Source: CAD feature listing. Evaluate the final solid. Frame: model axes, mm. Give positions to 0.01 mm unless a question says otherwise; leave off trailing zeros. Order: outer loops, then holes, each group sorted by start corner. A loop starts at its lowest first (then second) coordinate and runs counter-clockwise, first axis right, second up. Notation, with made-up numbers: (-14, 8.5) - (31, 8.5) arc R23 cw to (31, 43.5) - close; hole circle Ø1 at (-23, 60). An arc over 180 degrees is marked (long way). Answer as CSV lines item,"result".
```python
from build123d import *

# Parameters (mm, degrees)
SKETCH_1_R          = 1.621125
EXTRUDE_700_DEPTH   = 65
SKETCH_2_OUTSIDE_W  = 249.76
SKETCH_2_OUTSIDE_H  = 250.688
SKETCH_2_OUTSIDE_R  = 3
CUT_EXTRUDE_1_DEPTH = 66
CUT_EXTRUDE_1_TAPER = 60
SKETCH_3_OUTSIDE_W  = 249.76
SKETCH_3_OUTSIDE_H  = 250.688
SKETCH_3_OUTSIDE_R  = 3
CUT_EXTRUDE_2_DEPTH = 66
CUT_EXTRUDE_2_TAPER = 60


with BuildPart() as part:
    # 草图1 → Extrude 700 (new body)
    with BuildSketch(Plane.XY):
        Polygon((0, 3.464101615), (-3, 1.732050808), (-3, -1.732050808), (0, -3.464101615), (3, -1.732050808), (3, 1.732050808), align=None)
        Circle(SKETCH_1_R, mode=Mode.SUBTRACT)
    extrude(amount=EXTRUDE_700_DEPTH)

    # 草图2 outside → 切除-拉伸1 (cut, through all)
    with BuildSketch(Plane(origin=(0, 0, 0), x_dir=(-1, 0, 0), z_dir=(0, 0, -1))):
        Rectangle(SKETCH_2_OUTSIDE_W, SKETCH_2_OUTSIDE_H)
        Circle(SKETCH_2_OUTSIDE_R, mode=Mode.SUBTRACT)
    extrude(amount=-CUT_EXTRUDE_1_DEPTH, taper=CUT_EXTRUDE_1_TAPER, mode=Mode.SUBTRACT)

    # 草图3 outside → 切除-拉伸2 (cut, through all)
    with BuildSketch(Plane.XY.offset(65)):
        Rectangle(SKETCH_3_OUTSIDE_W, SKETCH_3_OUTSIDE_H)
        Circle(SKETCH_3_OUTSIDE_R, mode=Mode.SUBTRACT)
    extrude(amount=-CUT_EXTRUDE_2_DEPTH, taper=CUT_EXTRUDE_2_TAPER, mode=Mode.SUBTRACT)


solid = part.part
```
(1) Mould query, pull axis X, two halves, no side actions, for faces 1 (the conical face through (-2.744, 1.575, 64.905)), 2 (the flat face through (1.3, -1.3, 65)), 3 (the cylindrical face through (-0.351, -1.583, 32.045)). Classes: released by +X, released by -X, zero draft, split by the parting line, or undercut.
Completed:
face 1,"released by -X"
face 2,"zero draft"
face 3,"undercut"
(2) Ray query, line 1 (Y direction, x = 0, z = 27); line 2 (Y direction, x = 0.25, z = 38); line 3 (X direction, y = 0.75, z = 40). Return the intervals inside material, ascending. Write a range as from..to.
Completed:
line 1,"-3.46..-1.62, 1.62..3.46"
line 2,"-3.32..-1.6, 1.6..3.32"
line 3,"-3..-1.44, 1.44..3"
(3) Cut plane A-A (z = 34). Return loops of the section in (x, y), then the cut area to 3 significant figures.
Completed:
outline,"(-3, -1.73) - (0, -3.46) - (3, -1.73) - (3, 1.73) - (0, 3.46) - (-3, 1.73) - close; hole circle Ø3.24 at (0, 0)"
area,"22.9 mm²"
